Autodesk Inventor part; units mm, degrees
ref_plane "YZ Plane" through (0, 0, 0) normal (1, 0, 0) x (0, 1, 0)
ref_plane "XZ Plane" through (0, 0, 0) normal (0, 1, 0) x (-1, 0, 0)
ref_plane "XY Plane" through (0, 0, 0) normal (0, 0, 1) x (1, 0, 0)
sketch "Sketch1" plane through (0, 0, 0) normal (0, 1, 0) x (-1, 0, 0)
  line L0 (97.5, -33) -> (-97.5, -33)
  line L1 (-97.5, -33) -> (-97.5, 33)
  line L2 (-97.5, 33) -> (97.5, 33)
  line L3 (97.5, 33) -> (97.5, -33)
  line L4 (97.5, -33) -> (-97.5, 33) construction
  line L5 (-97.5, -33) -> (97.5, 33) construction
  point P0 (0, 0)
  dimension "d0" = 195
  dimension "d1" = 66
extrude "Extrusion1" add sketch "Sketch1" along normal blind 7
fillet "Fillet1" radius 2 4 edges at (-97.5, 3.5, 33) (97.5, 3.5, 33) (97.5, 3.5, -33) (-97.5, 3.5, -33)
sketch "Sketch2" plane through (0, 7, 0) normal (0, 1, 0) x (1, 0, 0)
  line L0 (-32.5, 27.25) -> (-30.5, 27.25) construction
  line L1 (-32.5, 25.65) -> (-30.5, 25.65)
  line L2 (-30.5, 28.85) -> (-32.5, 28.85)
  arc A0 (-32.5, 28.85) -> (-32.5, 25.65) centre (-32.5, 27.25) ccw
  arc A1 (-30.5, 25.65) -> (-30.5, 28.85) centre (-30.5, 27.25) ccw
  circle A2 centre (-89.5, 27.25) radius 1.6
  line L3 (30.5, 27.25) -> (32.5, 27.25) construction
  line L4 (30.5, 25.65) -> (32.5, 25.65)
  line L5 (32.5, 28.85) -> (30.5, 28.85)
  arc A3 (30.5, 28.85) -> (30.5, 25.65) centre (30.5, 27.25) ccw
  arc A4 (32.5, 25.65) -> (32.5, 28.85) centre (32.5, 27.25) ccw
  line L6 (88.5, 27.25) -> (90.5, 27.25) construction
  line L7 (88.5, 25.65) -> (90.5, 25.65)
  line L8 (90.5, 28.85) -> (88.5, 28.85)
  arc A5 (88.5, 28.85) -> (88.5, 25.65) centre (88.5, 27.25) ccw
  arc A6 (90.5, 25.65) -> (90.5, 28.85) centre (90.5, 27.25) ccw
  line L9 (95.5, 33) -> (-95.5, 33)
  line L10 (-97.5, 31) -> (-97.5, -31)
  line L11 (97.5, -31) -> (97.5, 31)
  point P0 (0, 0)
  point P1 (-31.5, 27.25)
  point P2 (31.5, 27.25)
  point P3 (89.5, 27.25)
  dimension "d9" = 1
  dimension "d10" = 3.2
  dimension "d11" = 3.2
  dimension "d12" = 1
  dimension "d13" = 3.2
  dimension "d14" = 1
  dimension "d15" = 3.2
  dimension "d16" = 58
  dimension "d17" = 63
  dimension "d18" = 58
  dimension "d19" = 5.75
  dimension "d21" = 8
extrude "Extrusion2" cut sketch "Sketch2" against normal through all
mirror "Mirror1" about plane through (0, 0, 0) normal (0, 0, 1) of "Extrusion2"
sketch "Sketch3" plane through (0, 0, 0) normal (0, -1, 0) x (1, 0, 0)
  circle A0 centre (-89.5, -27.25) radius 1.6
  line L0 (-87.7679, -24.25) -> (-86.0359, -27.25)
  line L1 (-86.0359, -27.25) -> (-87.7679, -30.25)
  line L2 (-87.7679, -30.25) -> (-91.2321, -30.25)
  line L3 (-91.2321, -30.25) -> (-92.9641, -27.25)
  line L4 (-92.9641, -27.25) -> (-91.2321, -24.25)
  line L5 (-91.2321, -24.25) -> (-87.7679, -24.25)
  point P0 (0, 0)
  dimension "d24" = 3
extrude "Extrusion3" cut sketch "Sketch3" against normal blind 5
pattern_linear "Rectangular Pattern1" count 2 spacing 58 along (1, 0, 0) of "Extrusion3"
mirror "Mirror2" about plane through (0, 0, 0) normal (0, 0, 1) of "Extrusion3", "Rectangular Pattern1"
mirror "Mirror3" about plane through (0, 0, 0) normal (1, 0, 0) of "Extrusion3", "Rectangular Pattern1", "Mirror2"
CAD build for the part. Positions are in the model's coordinates, mm. A direction names the side the tool comes from. Give positions to 0.01 mm unless a question says otherwise; leave off trailing zeros. Put each result on its own line as item: value.
(1) Tool access for faces 3 (the flat face through (-91, 5, 26)), 4 (the cylindrical face through (-91.1, 6, -27.3)): list every direction of +Z, -Z, +X, -X, +Y, -Y with a clear straight run to the whole face (end or side of a thin tool).
Working result:
face 3: -Y
face 4: +Y, -Y
(2) Wall check: L1, parallel to Z at x = -89.5, y = 5.6; L2, parallel to X at y = 5.95, z = -27.25; L3, parallel to X at y = 3.25, z = -28. Give the ranges that are in metal, low to high.
Working result:
L1: -33 to -28.85, -25.65 to 25.65, 28.85 to 33
L2: -97.5 to -91.1, -87.9 to -34.1, -28.9 to 28.9, 34.1 to 86.9, 92.1 to 97.5
L3: -97.5 to -92.53, -86.47 to -34.53, -28.47 to 28.47, 34.53 to 86.47, 92.53 to 97.5
(3) Drop a flat-ended pin along its axis: pin 1 Ø1.8 at (x, z) = (-91, -28.5) entering from -Y. Give the stop position or say it passes through.
Working result:
pin 1: y = 5
(4) Pull direction Z, two halves, no side cores. Call faces 1 (the flat face through (-31, 2, 24.25)), 2 (the flat face through (97.5, 3, 0)): released by +Z, released by -Z, zero draft, split by the parting line, or undercut.
Working result:
face 1: undercut
face 2: zero draft
(5) Saw through at A-A (y = 2.75). Count the separate pieces of the cut face and the enclosed holes in it, then the cut area to 3 significant figures.
Working result:
separate pieces: 1
enclosed holes: 8
area: 12,600 mm^2
